Input: dimensioned drawing with shaded views. Units: mm. Origin: part minimum x, y, z. A direction names the side the tool comes from. Coordinates: 2 decimals unless noted, no trailing zeros. Write each loop counter-clockwise with the first axis right and the second up, starting at its lowest first coordinate (ties: lowest second). Pieces come first, ordered by that corner, then holes. Notation, with made-up numbers: (52.25, 23) -> (74.25, 23) arc R13 ccw to (74.25, 39) -> close; hole circle Ø7 at (0.25, 2.25). An arc over 180 degrees is marked (long way). One line per item, written item: value. Start each with the question number.
1. Access query for the marked faces 4 and 5. Directions: +Z, -Z, +X, -X, +Y, -Y. A direction counts if a zero-diameter tool reaches every point of the face in a straight line with its end or side. Return the directions, or none.
2. First-contact query: P1, Ø3, axis at y = 3.5, z = 3.5, coming from the -X side. Flat tip, straight axial feed; report the tip coordinate or a pass-through.
3. Section query C-C, the plane x = 0.55. Output: boundary loops of the cut face in (y, z), and give its area (3 significant figures).
4. Mould query, pull axis Y, two halves, no side actions, for the marked faces 1, 2 and 3. Classes: released by +Y, released by -Y, zero draft, split by the parting line, or undercut.
5. Line query: line 1 (Z direction, x = 0.75, y = 3.5); line 2 (X direction, y = 2.75, z = 2); line 3 (Y direction, x = 1.2, z = 4.5). Output: solid intervals per line, ascending.
6. Section query A-A, the plane z = 3.5. Output: boundary loops of the cut face in (x, y), and give its area (3 significant figures).
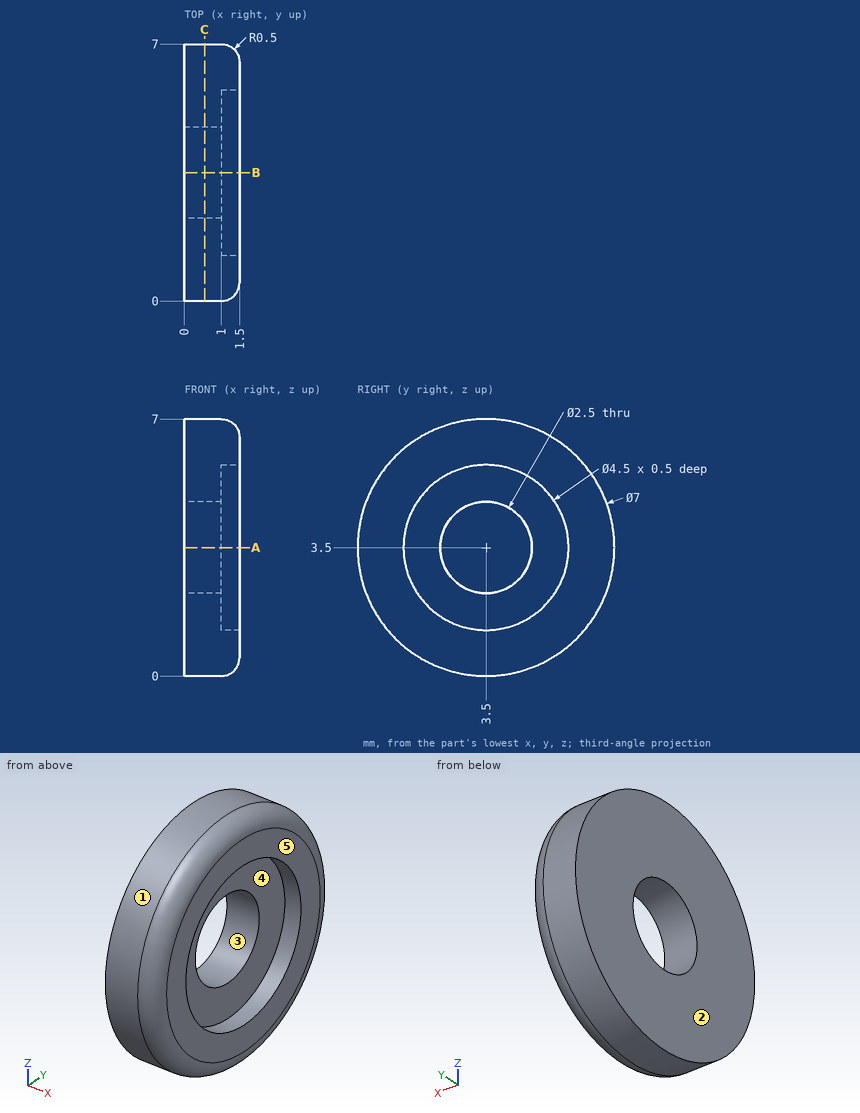
Computed values:
1. face 4: +X
1. face 5: +Z, -Z, +X, +Y, -Y
2. P1: stops at x = 0
3. outline: circle Ø7 at (3.5, 3.5); hole circle Ø2.5 at (3.5, 3.5)
3. area: 33.6 mm²
4. face 1: split by the parting line
4. face 2: zero draft
4. face 3: undercut
5. line 1: z = 0 to 2.25, 4.75 to 7
5. line 2: x = 0 to 1
5. line 3: y = 0.19 to 1.48, 5.52 to 6.81
6. outline: (0, 0) -> (1, 0) arc R0.5 ccw to (1.5, 0.5) -> (1.5, 1.25) -> (1, 1.25) -> (1, 2.25) -> (0, 2.25) -> close; (0, 4.75) -> (1, 4.75) -> (1, 5.75) -> (1.5, 5.75) -> (1.5, 6.5) arc R0.5 ccw to (1, 7) -> (0, 7) -> close
6. area: 5.64 mm²
